Can you work these out from the model? Positions are in its coordinate system, mm. Face numbers are marked on the shaded views. A direction names the side the tool comes from. Coordinates: 2 decimals unless noted, no trailing zeros. Loops run counter-clockwise (first coordinate to the right, second up) from the corner with the lowest first, then second, coordinate; pieces in that order, holes last. Notation, with made-up numbers: (28.25, 48.5) - (76.25, 48.5) arc R9 cw to (76.25, 58.5) - close; hole circle Ø8 at (31.25, -32). An arc over 180 degrees is marked (long way). Put each result on its own line as item: value. Start each with the question number.
Autodesk Inventor part; units mm, degrees
ref_plane "YZ Plane" through (0, 0, 0) normal (1, 0, 0) x (0, 1, 0)
ref_plane "XZ Plane" through (0, 0, 0) normal (0, 1, 0) x (-1, 0, 0)
ref_plane "XY Plane" through (0, 0, 0) normal (0, 0, 1) x (1, 0, 0)
sketch "Boceto1" plane through (0, 0, 0) normal (0, 0, 1) x (1, 0, 0)
  line L0 (0, 0) -> (33, 0)
  line L1 (33, 0) -> (33, 33)
  line L2 (33, 33) -> (0, 33)
  line L3 (0, 33) -> (0, 0)
  line L4 (10, 33) -> (30, 33)
  line L5 (30, 33) -> (30, 41)
  line L6 (30, 41) -> (10, 41)
  line L7 (10, 41) -> (10, 33)
  point P0 (30, 33)
  dimension "d4" = 33
  dimension "d5" = 33
  dimension "d6" = 41
  dimension "d7" = 3
  dimension "d8" = 10
extrude "Extrusión1" add sketch "Boceto1" along normal blind 40.5
sketch "Boceto2" plane through (10, 41, 0) normal (0, 1, 0) x (1, 0, 0)
  line L0 (20, -21) -> (0, -21)
  line L1 (0, -21) -> (0, -19.5)
  line L2 (0, -19.5) -> (20, -19.5)
  line L3 (20, -19.5) -> (20, -21)
  line L4 (0, 0) -> (0, -40.5)
  line L5 (20, 0) -> (20, -40.5)
  point P0 (-10, 0)
  point P1 (0, -20.25)
  point P2 (20, -20.25)
  dimension "d11" = 1.5
extrude "Extrusión2" add sketch "Boceto2" along normal blind 6
fillet "Empalme1" radius 0.2 6 edges at (10, 44, 21) (20, 47, 21) (30, 44, 21) (10, 44, 19.5) (20, 47, 19.5) (30, 44, 19.5)
sketch "Boceto3" plane through (10, 41, 40.5) normal (0, 1, 0) x (1, 0, 0)
  line L0 (0, 40.5) -> (0, 0)
  line L1 (0, 20.25) -> (20, 20.25)
  line L2 (20, 40.5) -> (20, 0)
  line L3 (10, 20.25) -> (10, 28.25)
  line L4 (10, 20.25) -> (10, 12.25)
  line L5 (19.8, 19.5) -> (0.2, 19.5)
  line L6 (10, 19.5) -> (12.8197, 19.5)
  line L7 (0.2, 21) -> (19.8, 21)
  line L8 (10, 21) -> (12.8197, 21)
  circle A0 centre (10, 12.25) radius 7.25
  circle A1 centre (10, 28.25) radius 7.25
  point P0 (-10, 40.5)
  dimension "d15" = 8
  dimension "d16" = 8
extrude "Extrusión3" add sketch "Boceto3" along normal blind 0.5
sketch "Boceto4" plane through (0, 0, 0) normal (0, -1, 0) x (1, 0, 0)
  line L0 (0, 0) -> (33, 0)
  line L1 (16.5, 0) -> (16.5, 40.5)
  line L2 (0, 40.5) -> (33, 40.5)
  line L3 (16.5, 20.25) -> (16.5, 48.25)
  circle A0 centre (16.5, 48.25) radius 3.2
  circle A1 centre (16.5, 48.25) radius 4
  line L4 (16.5, 40.5) -> (6.5, 40.5)
  line L5 (16.5, 40.5) -> (26.5, 40.5)
  line L6 (26.5, 40.5) -> (19.8242, 50.4748)
  line L7 (6.5, 40.5) -> (13.1758, 50.4748)
  line L8 (16.5, 20.25) -> (16.5, -7.75)
  circle A2 centre (16.5, -7.75) radius 3.2
  circle A3 centre (16.5, -7.75) radius 4
  line L9 (6.5, 0) -> (26.5, 0)
  line L10 (6.5, 0) -> (13.1758, -9.9748)
  line L11 (26.5, 0) -> (19.8242, -9.9748)
  dimension "d19" = 28
  dimension "d20" = 6.4
  dimension "d21" = 8
  dimension "d22" = 10
  dimension "d23" = 10
  dimension "d26" = 28
  dimension "d27" = 6.4
  dimension "d28" = 8
  dimension "d29" = 20
  dimension "d30" = 6.5
extrude "Extrusión4" add sketch "Boceto4" against normal blind 5.6
equation "\"d4\" = DistA"
equation "\"d5\" = DistC"
equation "\"d6\" = DistB"
equation "\"d9\" = DistEXT"
equation "\"d12\" = DistEXT2"
equation "\"d24\" = DistEXT3"
equation "\"DistA\" = 33"
equation "\"DistB\" = 41"
equation "\"DistEXT\" = 40.5"
equation "\"DistC\" = 33"
equation "\"DistEXT2\" = 6"
equation "\"DistEXT3\" = 5.6"
properties part number "Pieza3-Tarea2"
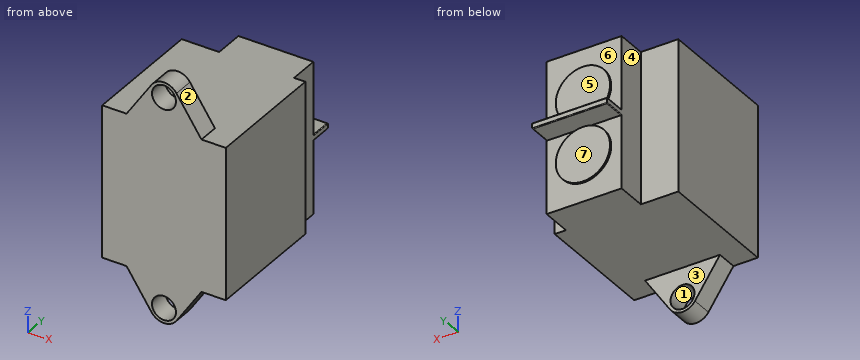
Q1. I want a section at B-B on x = 16.5. Count the separate pieces of the cut face and the enclosed holes in it, and give its area (3 significant figures).
Q2. On a 3-axis mill with a long thin cutter (end or side, diameter ignored), from which of +Z, -Z, +X, -X, +Y, -Y can I reach the whole of each face in a straight line? I mean the marked faces 4, 5, 6 and 7. Say none if no direction works.
Q3. Will these pins go through, and if not, where does the flat tip stop? pin 1 (10 mm diameter, centred on x = 24.5, y = 30, fed in from -Z); pin 2 (15.5 mm diameter, centred on y = 41.5, z = 28, fed in from +X); pin 3 (9.5 mm diameter, centred on x = 19, z = -7.5, fed in from +Y).
Q4. I want a section at D-D on y = 21. List the corners of the cut face in (x, z) for me, and give its area (3 significant figures).
Q5. Please list where these lines run through material, in increasing order: line 1 along Z through (x, y) = (16.5, 4.1); line 2 along Y through (x, z) = (15, 14); line 3 along Y through (x, z) = (21.5, 43). Write a range as [from, to].
Q6. I want a section at C-C on z = 46.5. List the corners of the cut face in (x, y) for me, and give its area (3 significant figures).
Q7. I want a section at A-A on z = 28.25. List the corners of the cut face in (x, y) for me, and give its area (3 significant figures).
Q8. We'd pull the mould along X, two halves only. Please class the marked faces 1, 2 and 3: released by +X, released by -X, zero draft, split by the parting line, or undercut.
Calculated:
1. separate pieces: 3
1. enclosed holes: 0
1. area: 1,740 mm2
2. face 4: +Z, -Z, -X, +Y
2. face 5: +Z, +X, -X, +Y
2. face 6: +Y
2. face 7: -Z, +X, -X, +Y
3. pin 1: z = 0
3. pin 2: x = 30
3. pin 3: y = 5.6
4. outline: (0, 0) - (33, 0) - (33, 40.5) - (0, 40.5) - close
4. area: 1,340 mm2
5. line 1: [-11.75, -10.95], [-4.55, 45.05], [51.45, 52.25]
5. line 2: [0, 41.5]
5. line 3: [0, 5.6]
6. outline: (10.52, 0) - (13.82, 0) - (13.82, 5.6) - (10.52, 5.6) - close; (19.18, 0) - (22.48, 0) - (22.48, 5.6) - (19.18, 5.6) - close
6. area: 37.0 mm2
7. outline: (0, 0) - (33, 0) - (33, 33) - (30, 33) - (30, 41) - (27.25, 41) - (27.25, 41.5) - (12.75, 41.5) - (12.75, 41) - (10, 41) - (10, 33) - (0, 33) - close
7. area: 1,260 mm2
8. face 1: undercut
8. face 2: released by +X
8. face 3: zero draft
